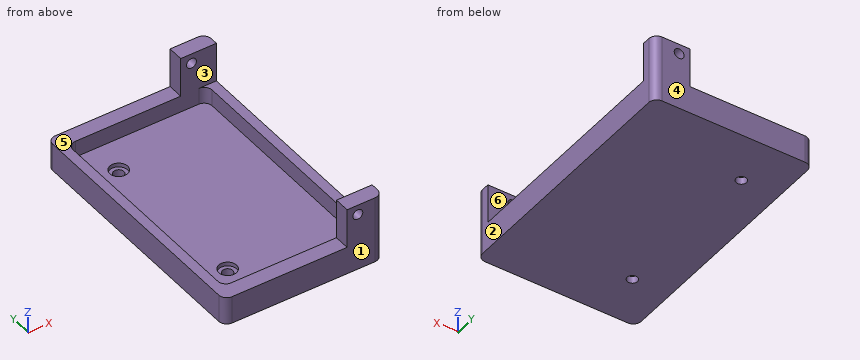
from build123d import *

# Parameters (mm, degrees)
F0_W      = 50.8
F0_H      = 82.55
F1_DEPTH  = 8.89
F2_W      = 44.577
F2_H      = 72.644
F3_DEPTH  = 5.334
F4_R      = 2.54
F5_R      = 1.651
F6_DEPTH  = 25.4
F7_R      = 2.8575
F8_DEPTH  = 1.27
F9_W      = 11.43
F9_H      = 4.953
F10_DEPTH = 12.7
F11_R     = 1.5875
F12_DEPTH = 127
F13_R     = 2.54


with BuildPart() as f1:
    # F0 (on Top) → F1 (new body)
    with BuildSketch(Plane.XY):
        with Locations((-5.138001, -3.863245)):
            Rectangle(F0_W, F0_H)
    extrude(amount=F1_DEPTH)

    # F2 (on face) → F3 (cut)
    with BuildSketch(Plane.XY.offset(8.89)):
        with Locations((-5.138001, -3.863245)):
            Rectangle(F2_W, F2_H)
    extrude(amount=-F3_DEPTH, mode=Mode.SUBTRACT)

    # F4
    f4_edges = [f1.edges().sort_by_distance(p)[0] for p in [
        (-27.426501, 32.458755, 6.223),
        (17.150499, 32.458755, 6.223),
        (17.150499, -40.185245, 6.223),
        (-27.426501, -40.185245, 6.223),
    ]]
    fillet(f4_edges, radius=F4_R)

    # F5 (on face) → F6 (cut)
    with BuildSketch(Plane.XY.offset(3.556)):
        with Locations((-18.536501, 21.536755)):
            Circle(F5_R)
        with Locations((-18.536501, -29.263245)):
            Circle(F5_R)
    extrude(amount=-F6_DEPTH, mode=Mode.SUBTRACT)

    # F7 (on face) → F8 (cut)
    with BuildSketch(Plane.XY.offset(3.556)):
        with Locations((-18.536501, 21.536755)):
            Circle(F7_R)
        with Locations((-18.536501, -29.263245)):
            Circle(F7_R)
    extrude(amount=-F8_DEPTH, mode=Mode.SUBTRACT)

    # F9 (on face) → F10 (join)
    with BuildSketch(Plane.XY.offset(8.89)):
        with Locations((14.546999, -42.661745)):
            Rectangle(F9_W, F9_H)
        with Locations((14.546999, 34.935255)):
            Rectangle(F9_W, F9_H)
    extrude(amount=F10_DEPTH)

    # F11 (on face) → F12 (cut)
    with BuildSketch(Plane.XZ.offset(45.138245)):
        with Locations((12.260999, 18.444914)):
            Circle(F11_R)
    extrude(amount=-F12_DEPTH, mode=Mode.SUBTRACT)

    # F13
    f13_edges = [f1.edges().sort_by_distance(p)[0] for p in [
        (20.261999, -45.138245, 10.795),
        (-30.538001, -45.138245, 4.445),
        (20.261999, 37.411755, 10.795),
        (-30.538001, 37.411755, 4.445),
    ]]
    fillet(f13_edges, radius=F13_R)


solid = f1.part
Part model, mm, in its own coordinate system. Face numbers are marked on the shaded views. A direction names the side the tool comes from. Coordinates: 2 decimals unless noted, no trailing zeros. Order: outer loops, then holes, each group sorted by start corner. A loop starts at its lowest first (then second) coordinate and runs counter-clockwise, first axis right, second up. Notation, with made-up numbers: M -10.75,85 L 9.25,85 A34 cw 9.25,121 Z; hole C 39,61 d2. An arc over 180 degrees is marked long. Use a Markdown table: item, result.
(1) Cut at B-B on z = 5. Write the cut outline in (x, y).
A:
| item | result |
|---|---|
| outline | M -30.54,-42.6 A2.54 ccw -28,-45.14 L 17.72,-45.14 A2.54 ccw 20.26,-42.6 L 20.26,34.87 A2.54 ccw 17.72,37.41 L -28,37.41 A2.54 ccw -30.54,34.87 Z; hole M -27.43,-37.65 A2.54 ccw -24.89,-40.19 L 14.61,-40.19 A2.54 ccw 17.15,-37.65 L 17.15,29.92 A2.54 ccw 14.61,32.46 L -24.89,32.46 A2.54 ccw -27.43,29.92 Z |
(2) Tool access for the marked faces 4, 5 and 6: list every direction of +Z, -Z, +X, -X, +Y, -Y with a clear straight run to the whole face (end or side of a thin tool).
A:
| item | result |
|---|---|
| face 4 | +Z, -Z, +X, -X, +Y |
| face 5 | +Z, -X, +Y, -Y |
| face 6 | +Z |
(3) Flat gauge pins, fed straight in: pin 1 (6 mm diameter, centred on x = 8.5, z = 12, fed in from +Y); pin 2 (2 mm diameter, centred on x = 1.5, y = -25, fed in from +Z); pin 3 (4.5 mm diameter, centred on x = 18, y = -17, fed in from +Z); pin 4 (5 mm diameter, centred on x = -18.54, y = -29.26, fed in from +Z). Where does each tip first touch, or does it go through?
A:
| item | result |
|---|---|
| pin 1 | stops at y = 37.41 |
| pin 2 | stops at z = 3.56 |
| pin 3 | stops at z = 8.89 |
| pin 4 | stops at z = 2.29 |
(4) Cut at A-A on z = 14.25. Write the cut outline in (x, y), then the cut area to 3 significant figures.
A:
| item | result |
|---|---|
| outline | M 8.83,-45.14 L 17.72,-45.14 A2.54 ccw 20.26,-42.6 L 20.26,-40.19 L 8.83,-40.19 Z; M 8.83,32.46 L 20.26,32.46 L 20.26,34.87 A2.54 ccw 17.72,37.41 L 8.83,37.41 Z |
| area | 110 mm^2 |
(5) Cut at C-C on y = 11. Write the cut outline in (x, z).
A:
| item | result |
|---|---|
| outline | M -30.54,0 L 20.26,0 L 20.26,8.89 L 17.15,8.89 L 17.15,3.56 L -27.43,3.56 L -27.43,8.89 L -30.54,8.89 Z |
(6) Pull direction X, two halves, no side cores. Call the marked faces 1, 2 and 3: released by +X, released by -X, zero draft, split by the parting line, or undercut.
A:
| item | result |
|---|---|
| face 1 | zero draft |
| face 2 | released by +X |
| face 3 | undercut |
(7) Probe L1, parallel to Y at x = -18, z = 4.25; L2, parallel to X at y = 25.5, z = 5; L3, parallel to Z at x = 2, y = 12. List the from-to ranges inside material, lowest first.
A:
| item | result |
|---|---|
| L1 | y = -45.14 to -40.19, 32.46 to 37.41 |
| L2 | x = -30.54 to -27.43, 17.15 to 20.26 |
| L3 | z = 0 to 3.56 |
(8) Cut at D-D on x = 0. Write the cut outline in (y, z), then the cut area to 3 significant figures.
A:
| item | result |
|---|---|
| outline | M -45.14,0 L 37.41,0 L 37.41,8.89 L 32.46,8.89 L 32.46,3.56 L -40.19,3.56 L -40.19,8.89 L -45.14,8.89 Z |
| area | 346 mm^2 |
